Geometry: final body of the model. Coordinates: model frame, mm. A direction names the side the tool comes from. Give positions to 0.01 mm unless a question says otherwise; leave off trailing zeros. Write each loop counter-clockwise with the first axis right and the second up, starting at its lowest first coordinate (ties: lowest second). Pieces come first, ordered by that corner, then holes. Notation, with made-up numbers: (26.25, 16) -> (62.25, 16) arc R17 ccw to (62.25, 47) -> close; hole circle Ø8 at (15, -14.5). An arc over 180 degrees is marked (long way). Answer in a Markdown table with one row per item. Add a question column.
Item 1: First-contact query: P1, Ø9.5, axis at x = 70, z = -35, coming from the +Y side; P2, Ø0.8, axis at y = 2.5, z = 15, coming from the -X side. Flat tips, straight axial feed; report the tip coordinate or a pass-through.
Item 2: Section query C-C on y = 2.8. Output: boundary loops of the cut face in (x, z), plus the area to 3 significant figures.
Item 3: Section query D-D on x = 33.5. Output: boundary loops of the cut face in (y, z).
Item 4: Section query B-B on z = -25. Output: boundary loops of the cut face in (x, y).
Item 5: Access query for faces 1 (the flat face through (-1, 2, -1)), 2 (the cylindrical face through (68.2, 1, 32.6)). Directions: +Z, -Z, +X, -X, +Y, -Y. A direction counts if a zero-diameter tool reaches every point of the face in a straight line with its end or side. Return the directions, or none.
Item 6: Draft query along Z for faces 3 (the cylindrical face through (-71.8, 1, -37.4)), 4 (the flat face through (-1, 0, -1)). Return one class per face: +Z half, -Z half, draft (parallel to the pull), parting line (faces both ways), or undercut.
Item 7: Section query A-A on x = -70. Output: boundary loops of the cut face in (y, z).
Item 8: Material intervals for probe 1 along X at (y, z) = (1.5, -35); probe 2 along Y at (x, z) = (21, 30); probe 3 along X at (y, z) = (3.2, 22), sorted ascending. Write a range as from..to.
```python
from build123d import *

# Parameters (mm, degrees)
SKETCH1_W               = 160
SKETCH1_H               = 90
BOSS_EXTRUDE1_DEPTH     = 2
BOSS_EXTRUDE2_DEPTH     = 90
BOSS_EXTRUDE5_DEPTH     = 164
CUT_EXTRUDE1_DEPTH      = 164
CUT_EXTRUDE1_DEPTH_BACK = 164
SKETCH5_R               = 3
CUT_EXTRUDE2_DEPTH      = 164


with BuildPart() as part:
    # Sketch1 → Boss-Extrude1 (new body)
    with BuildSketch(Plane(origin=(0, 0, 0), x_dir=(1, 0, 0), z_dir=(0, 1, 0))):
        Rectangle(SKETCH1_W, SKETCH1_H)
    extrude(amount=BOSS_EXTRUDE1_DEPTH)

    # Sketch2 → Boss-Extrude2 (add)
    with BuildSketch(Plane.XY.offset(45)):
        Polygon((-82, 0), (-80, 0), (-80, 3.5), (-82, 2), align=None)
        Polygon((80, 0), (82, 0), (82, 2), (80, 3.5), align=None)
    extrude(amount=-BOSS_EXTRUDE2_DEPTH)

    # Sketch3 → Boss-Extrude5 (add)
    with BuildSketch(Plane.ZY.offset(82)):
        Polygon((-47, 0), (-45, 0), (-45, 3.5), (-47, 2), align=None)
        Polygon((45, 0), (45, 3.5), (47, 2), (47, 0), align=None)
    extrude(amount=-BOSS_EXTRUDE5_DEPTH)

    # Sketch4 → Cut-Extrude1 (cut, two sides: drawn at the far end of the back side and taken through both)
    with BuildSketch(Plane.XY.offset(-45).offset(-CUT_EXTRUDE1_DEPTH_BACK)):
        Polygon((-80, 3.5), (-82, 2), (-82, 3.5), align=None)
        Polygon((80, 3.5), (82, 3.5), (82, 2), align=None)
    extrude(amount=CUT_EXTRUDE1_DEPTH + CUT_EXTRUDE1_DEPTH_BACK, mode=Mode.SUBTRACT)

    # Sketch5 → Cut-Extrude2 (cut)
    with BuildSketch(Plane(origin=(0, 2, 0), x_dir=(1, 0, 0), z_dir=(0, 1, 0))):
        with Locations(Location((-70, 35, 0), (0, 0, 270))):
            Circle(SKETCH5_R)
        with Locations(Location((70, 35, 0), (0, 0, 270))):
            Circle(SKETCH5_R)
        with Locations(Location((70, -35, 0), (0, 0, 270))):
            Circle(SKETCH5_R)
        with Locations(Location((-70, -35, 0), (0, 0, 270))):
            Circle(SKETCH5_R)
    extrude(amount=-CUT_EXTRUDE2_DEPTH, mode=Mode.SUBTRACT)


solid = part.part
```
Findings below:
| question | item | result |
|---|---|---|
| 1 | P1 | stops at y = 2 |
| 1 | P2 | stops at x = -81.87 |
| 2 | outline | (-80.93, -45.93) -> (80.93, -45.93) -> (80.93, 45.93) -> (-80.93, 45.93) -> close; hole (-80, -45) -> (80, -45) -> (80, 45) -> (-80, 45) -> close |
| 2 | area | 470 mm^2 |
| 3 | outline | (0, -47) -> (2, -47) -> (3.5, -45) -> (2, -45) -> (2, 45) -> (3.5, 45) -> (2, 47) -> (0, 47) -> close |
| 4 | outline | (-82, 0) -> (82, 0) -> (82, 2) -> (80, 3.5) -> (80, 2) -> (-80, 2) -> (-80, 3.5) -> (-82, 2) -> close |
| 5 | face 1 | +Y |
| 5 | face 2 | +Y, -Y |
| 6 | face 3 | undercut |
| 6 | face 4 | draft |
| 7 | outline | (0, -47) -> (2, -47) -> (3.5, -45) -> (2, -45) -> (2, -38) -> (0, -38) -> close; (0, -32) -> (2, -32) -> (2, 32) -> (0, 32) -> close; (0, 38) -> (2, 38) -> (2, 45) -> (3.5, 45) -> (2, 47) -> (0, 47) -> close |
| 8 | probe 1 | x = -82..-73, -67..67, 73..82 |
| 8 | probe 2 | y = 0..2 |
| 8 | probe 3 | x = -80.4..-80, 80..80.4 |
